Design review of the part built by this model. Coordinates are the model's own, in mm. A direction names the side the tool comes from. Coordinates: 2 decimals unless noted, no trailing zeros. Loops run counter-clockwise (first coordinate to the right, second up) from the corner with the lowest first, then second, coordinate; pieces in that order, holes last. Notation, with made-up numbers: M -36.75,83 L -32.75,83 A21 ccw -32.75,122 Z; hole C -19.5,0.5 d11. An arc over 180 degrees is marked long. One line per item, written item: value.
```python
from build123d import *

# Parameters (mm, degrees)
SKETCH_1_W          = 20
SKETCH_1_H          = 20
EXTRUDE_1_DEPTH     = 4
SKETCH_2_W          = 12.9
SKETCH_2_H          = 20
EXTRUDE_2_DEPTH     = 4.5
SKETCH_3_R          = 1.6
CUT_EXTRUDE_1_DEPTH = 30.533878851
SKETCH_4_W          = 5.8
SKETCH_4_H          = 20
SKETCH_4_R          = 1.6
EXTRUDE_3_DEPTH     = 2
SKETCH_5_R          = 3
CUT_EXTRUDE_3_DEPTH = 2.4
CHAMFER_3_SIZE      = 1.5
CHAMFER_1_SIZE      = 6.6
CHAMFER_2_SIZE      = 1
CHAMFER_4_SIZE      = 0.4
CHAMFER_5_SIZE      = 0.9


with BuildPart() as part:
    # 草图1 → 凸台-拉伸1 (new body)
    with BuildSketch(Plane(origin=(0, 0, 0), x_dir=(1, 0, 0), z_dir=(0, 1, 0))):
        with Locations((10, 10)):
            Rectangle(SKETCH_1_W, SKETCH_1_H)
    extrude(amount=EXTRUDE_1_DEPTH)

    # 草图2 → 凸台-拉伸2 (add)
    with BuildSketch(Plane(origin=(0, 4, 0), x_dir=(1, 0, 0), z_dir=(0, 1, 0))):
        with Locations((6.45, 10)):
            Rectangle(SKETCH_2_W, SKETCH_2_H)
    extrude(amount=EXTRUDE_2_DEPTH)

    # 草图3 → 切除-拉伸1 (cut, through all)
    with BuildSketch(Plane(origin=(0, 0, 0), x_dir=(-1, 0, 0), z_dir=(0, -1, 0))):
        with Locations(Location((-10, 5, 0), (0, 0, 90))):
            Circle(SKETCH_3_R)
        with Locations(Location((-10, 15, 0), (0, 0, 90))):
            Circle(SKETCH_3_R)
    extrude(amount=-CUT_EXTRUDE_1_DEPTH, mode=Mode.SUBTRACT)

    # 草图4 → 凸台-拉伸3 (add)
    with BuildSketch(Plane(origin=(0, 8.5, 0), x_dir=(1, 0, 0), z_dir=(0, 1, 0))):
        with Locations((10, 10)):
            Rectangle(SKETCH_4_W, SKETCH_4_H)
        with Locations(Location((10, 15, 0), (0, 0, 90))):
            Circle(SKETCH_4_R, mode=Mode.SUBTRACT)
        with Locations(Location((10, 5, 0), (0, 0, 90))):
            Circle(SKETCH_4_R, mode=Mode.SUBTRACT)
    extrude(amount=EXTRUDE_3_DEPTH)

    # 草图5 → 切除-拉伸3 (cut)
    with BuildSketch(Plane(origin=(0, 0, 0), x_dir=(-1, 0, 0), z_dir=(0, -1, 0))):
        with Locations(Location((-10, 5, 0), (0, 0, 90))):
            Circle(SKETCH_5_R)
        with Locations(Location((-10, 15, 0), (0, 0, 90))):
            Circle(SKETCH_5_R)
    extrude(amount=-CUT_EXTRUDE_3_DEPTH, mode=Mode.SUBTRACT)

    # 倒角3
    # the kernel refuses this chamfer: 1.5 mm, written as the material it takes off along each edge
    with BuildSketch(Plane(origin=(10, 2.4, -15), x_dir=(0, 0, -1), z_dir=(-1, 0, 0))) as chamfer_3_piece_1_section:
        Polygon((1.6 + CHAMFER_3_SIZE, 0), (1.6, -CHAMFER_3_SIZE), (1.6, 0), align=None)
    chamfer_3_piece_1 = revolve(axis=Axis((10, 2.4, -15), (0, -1, 0)), mode=Mode.PRIVATE)
    chamfer_3_piece_1 = chamfer_3_piece_1 & Plane(origin=(10, 3.20338318, -15), x_dir=(0, 0, -1), z_dir=(0, -1, 0)) * Cylinder(3, 13, mode=Mode.PRIVATE)
    add(chamfer_3_piece_1, mode=Mode.SUBTRACT)
    with BuildSketch(Plane(origin=(10, 2.4, -5), x_dir=(0, 0, -1), z_dir=(-1, 0, 0))) as chamfer_3_piece_2_section:
        Polygon((1.6 + CHAMFER_3_SIZE, 0), (1.6, -CHAMFER_3_SIZE), (1.6, 0), align=None)
    chamfer_3_piece_2 = revolve(axis=Axis((10, 2.4, -5), (0, -1, 0)), mode=Mode.PRIVATE)
    chamfer_3_piece_2 = chamfer_3_piece_2 & Plane(origin=(10, 3.20338318, -5), x_dir=(0, 0, -1), z_dir=(0, -1, 0)) * Cylinder(3, 13, mode=Mode.PRIVATE)
    add(chamfer_3_piece_2, mode=Mode.SUBTRACT)

    # 倒角1
    chamfer_1_edges = [part.edges().sort_by_distance(p)[0] for p in [
        (0, 0, -10),
    ]]
    chamfer(chamfer_1_edges, length=CHAMFER_1_SIZE)

    # 倒角2
    chamfer_2_edges = [part.edges().sort_by_distance(p)[0] for p in [
        (20, 4, -10),
        (16.45, 4, 0),
        (12.9, 7.25, 0),
        (12.9, 7.25, -20),
        (16.45, 4, -20),
        (20, 0, -10),
    ]]
    chamfer(chamfer_2_edges, length=CHAMFER_2_SIZE)

    # 倒角4
    chamfer_4_edges = [part.edges().sort_by_distance(p)[0] for p in [
        (0, 8.5, -10),
    ]]
    chamfer(chamfer_4_edges, length=CHAMFER_4_SIZE)

    # 倒角5
    chamfer_5_edges = [part.edges().sort_by_distance(p)[0] for p in [
        (7.1, 10.5, -10),
        (12.9, 10.5, -10),
    ]]
    chamfer(chamfer_5_edges, length=CHAMFER_5_SIZE)


solid = part.part
```
(1) We need section D-D on z = -18.5. State the section outline as (x, y) points, then the cut area to 3 significant figures.
Reply:
outline: M 0,6.6 L 6.6,0 L 19,0 L 20,1 L 20,3 L 19,4 L 12.9,4 L 12.9,9.6 L 12,10.5 L 8,10.5 L 7.1,9.6 L 7.1,8.5 L 0.4,8.5 L 0,8.1 Z
area: 126 mm2
(2) We need section B-B on z = -15. State the section outline as (x, y) points, then the cut area to 3 significant figures.
Reply:
outline: M 0,6.6 L 6.6,0 L 7,0 L 7,2.5 L 8.4,3.9 L 8.4,10.5 L 8,10.5 L 7.1,9.6 L 7.1,8.5 L 0.4,8.5 L 0,8.1 Z; M 11.6,3.9 L 13,2.5 L 13,0 L 19,0 L 20,1 L 20,3 L 19,4 L 12.9,4 L 12.9,9.6 L 12,10.5 L 11.6,10.5 Z
area: 83.4 mm2
(3) Mouldability with a two-part tool opening along Z and no side actions: class faces 1 (the flat face through (12.9, 7, -10)), 2 (the cylindrical face through (10, 1, -2)), 3 (the flat face through (10, 4, 0)) as released by +Z, released by -Z, zero draft, split by the parting line, or undercut.
Reply:
face 1: zero draft
face 2: undercut
face 3: released by +Z
(4) To check wall thickness, follow line 1 along Z through (x, y) = (10, 7.5); line 2 along X through (y, z) = (7.5, -11); line 3 along Y through (x, z) = (15.25, -12). State the ranges of each line that lie inside material, in increasing order. Write a range as [from, to].
Reply:
line 1: z = [-20, -16.6], [-13.4, -6.6], [-3.4, 0]
line 2: x = [0, 12.9]
line 3: y = [0, 4]
(5) We need section C-C on y = 7. State the section outline as (x, z) points, then the cut area to 3 significant figures.
Reply:
outline: M 0,-20 L 11.9,-20 L 12.9,-19 L 12.9,-1 L 11.9,0 L 0,0 Z; hole C 10,-15 d3.2; hole C 10,-5 d3.2
area: 241 mm2
(6) Insertion check: pin 1 (6.5 mm diameter, centred on x = 16, z = -9.5, fed in from +Y); pin 2 (3 mm diameter, centred on y = 6, z = -9.5, fed in from +X); pin 3 (0.9 mm diameter, centred on y = 9, z = -14, fed in from -X); pin 4 (3 mm diameter, centred on x = 10, z = -15, fed in from +Y). Each pin has a flat end and moves straight along its axis. Give the tip position at first contact, or say it passes through.
Reply:
pin 1: stops at y = 9.75
pin 2: stops at x = 12.9
pin 3: stops at x = 7.1
pin 4: passes through
(7) Tool access review of faces 4 (the flat face through (12.4, 6.8, -19.5)), 5 (the flat face through (15.9, 3.5, -0.5)), 6 (the flat face through (16, 4, -10)), 7 (the cylindrical face through (10, 1, -12)): name each direction out of +Z, -Z, +X, -X, +Y, -Y from which nothing blocks a thin tool from reaching the whole face with its end or side.
Reply:
face 4: -Z, +X, +Y
face 5: +Z, +X, +Y
face 6: +Z, -Z, +X, +Y
face 7: -Y
(8) We need section A-A on x = 10. State the section outline as (y, z) points.
Reply:
outline: M 0,-20 L 10.5,-20 L 10.5,-16.6 L 3.9,-16.6 L 2.5,-18 L 0,-18 Z; M 0,-12 L 2.5,-12 L 3.9,-13.4 L 10.5,-13.4 L 10.5,-6.6 L 3.9,-6.6 L 2.5,-8 L 0,-8 Z; M 0,-2 L 2.5,-2 L 3.9,-3.4 L 10.5,-3.4 L 10.5,0 L 0,0 Z
